from build123d import *

# Parameters (mm, degrees)
EXTRUDE_1_DEPTH = 3.5
EXTRUDE_2_DEPTH = 0.5
EXTRUDE_3_DEPTH = 0.7
SKETCH_4_R      = 2.25
EXTRUDE_4_DEPTH = 0.3
EXTRUDE_5_DEPTH = 1


with BuildPart() as part:
    # 草图1 → 凸台-拉伸1 (new body)
    with BuildSketch(Plane(origin=(0, 0, 0), x_dir=(1, 0, 0), z_dir=(0, 1, 0))):
        Polygon((0, 4.902463921), (0, 1.097536079), (0.55, 0.547536079), (1.097536079, 0), (4.902463921, 0), (5.45, 0.547536079), (6, 1.097536079), (6, 4.902463921), (5.45, 5.452463921), (4.902463921, 6), (1.097536079, 6), (0.55, 5.452463921), align=None)
    extrude(amount=EXTRUDE_1_DEPTH)

    # 草图2 → 凸台-拉伸2 (add)
    with BuildSketch(Plane(origin=(0, 3.5, 0), x_dir=(1, 0, 0), z_dir=(0, 1, 0))):
        Polygon((1.30464286, 5.5), (4.69535714, 5.5), (5.5, 4.69535714), (5.5, 1.30464286), (4.69535714, 0.5), (1.30464286, 0.5), (0.5, 1.30464286), (0.5, 4.69535714), align=None)
    extrude(amount=EXTRUDE_2_DEPTH)

    # 草图3 → 凸台-拉伸3 (add)
    with BuildSketch(Plane(origin=(0, 4, 0), x_dir=(1, 0, 0), z_dir=(0, 1, 0))):
        Polygon((4.591803749, 5.25), (1.408196251, 5.25), (0.75, 4.591803749), (0.75, 1.408196251), (1.408196251, 0.75), (4.591803749, 0.75), (5.25, 1.408196251), (5.25, 4.591803749), align=None)
    extrude(amount=EXTRUDE_3_DEPTH)

    # 草图4 → 凸台-拉伸4 (add)
    with BuildSketch(Plane(origin=(0, 4.7, 0), x_dir=(1, 0, 0), z_dir=(0, 1, 0))):
        with Locations(Location((3, 3, 0), (0, 0, 270))):
            Circle(SKETCH_4_R)
    extrude(amount=EXTRUDE_4_DEPTH)

    # 放样2: read off the stored shape, not the designer's step
    # 放样2: loft between two sections, ruled curve by curve
    loft_2_from = [
        Edge.make_line((1.408196251, 4.7, -5.25), (0.75, 4.7, -4.591803749)),
        Edge.make_line((5.25, 4.7, -4.591803749), (4.591803749, 4.7, -5.25)),
        Edge.make_line((4.591803749, 4.7, -0.75), (5.25, 4.7, -1.408196251)),
        Edge.make_line((0.75, 4.7, -1.408196251), (1.408196251, 4.7, -0.75)),
        Edge.make_line((4.591803749, 4.7, -5.25), (1.408196251, 4.7, -5.25)),
        Edge.make_line((5.25, 4.7, -1.408196251), (5.25, 4.7, -4.591803749)),
        Edge.make_line((0.75, 4.7, -1.408196251), (0.75, 4.7, -4.591803749)),
        Edge.make_line((1.408196251, 4.7, -0.75), (4.591803749, 4.7, -0.75)),
    ]
    loft_2_to = [
        Edge.make_line((1.30464286, 4, -5.5), (0.5, 4, -4.69535714)),
        Edge.make_line((5.5, 4, -4.69535714), (4.69535714, 4, -5.5)),
        Edge.make_line((4.69535714, 4, -0.5), (5.5, 4, -1.30464286)),
        Edge.make_line((0.5, 4, -1.30464286), (1.30464286, 4, -0.5)),
        Edge.make_line((4.69535714, 4, -5.5), (1.30464286, 4, -5.5)),
        Edge.make_line((5.5, 4, -1.30464286), (5.5, 4, -4.69535714)),
        Edge.make_line((0.5, 4, -1.30464286), (0.5, 4, -4.69535714)),
        Edge.make_line((1.30464286, 4, -0.5), (4.69535714, 4, -0.5)),
    ]
    loft_2 = Solid(Shell([*[Face.make_surface_from_curves(loft_2_from[k], loft_2_to[k]) for k in range(8)], Face(Wire(loft_2_from)), Face(Wire(loft_2_to))]))
    add(loft_2)

    # 草图5 → 凸台-拉伸5 (add)
    with BuildSketch(Plane.XZ):
        Polygon((0, -3), (0, -2.3), (-0.15, -2.3), (-0.15, -3.7), (0, -3.7), align=None)
        Polygon((6, -3), (6, -2.3), (6.15, -2.3), (6.15, -3.7), (6, -3.7), align=None)
    extrude(amount=-EXTRUDE_5_DEPTH)


solid = part.part
The listing builds one solid part. Answer for the finished solid, in the listing's coordinates (mm). A direction names the side the tool comes from. Give positions to 0.01 mm unless a question says otherwise; leave off trailing zeros. Write each loop counter-clockwise with the first axis right and the second up, starting at its lowest first coordinate (ties: lowest second). Pieces come first, ordered by that corner, then holes. Notation, with made-up numbers: (-22, 5) - (-10, 5) arc R24 cw to (-10, 43) - close; hole circle Ø1 at (71.5, 27.25). An arc over 180 degrees is marked (long way). Use a Markdown table: item, result.
1. A tool of negligible diameter and unlimited length cuts with its end or side. For faces 1 (the flat face through (0.908, 3.746, -0.897)), 2 (the flat face through (3.2, 3.5, -0.3)), 3 (the flat face through (4.7, 4.7, -4.8)), from which of +Z, -Z, +X, -X, +Y, -Y can it reach the whole face along a straight path? Write none if from no direction.
Values follow:
| item | result |
|---|---|
| face 1 | +Z, -X, +Y |
| face 2 | +Y |
| face 3 | -Z, +X, +Y |
2. Section B-B on x = 5.75 is taken. Write down the section's boundary in (y, z), plus the area to 3 significant figures.
Values follow:
| item | result |
|---|---|
| outline | (0, -5.15) - (3.5, -5.15) - (3.5, -0.85) - (0, -0.85) - close |
| area | 15.1 mm² |
3. This flat-tipped pin is pushed along its axis until it touches: P1, Ø3, axis at y = 3, z = -2, coming from the +X side. Where does it stop, or does it pass through?
Values follow:
| item | result |
|---|---|
| P1 | stops at x = 6 |
4. Find the intervals of material crossed by probe 1 along X at (y, z) = (3.7, -2.55); probe 2 along Y at (x, z) = (1.25, -4.6); probe 3 along X at (y, z) = (2.5, -4.45), in increasing order. Write a range as from..to.
Values follow:
| item | result |
|---|---|
| probe 1 | x = 0.5..5.5 |
| probe 2 | y = 0..4.7 |
| probe 3 | x = 0..6 |
5. Section A-A on y = 3.35 is taken. Write down the section's boundary in (x, z).
Values follow:
| item | result |
|---|---|
| outline | (0, -4.9) - (1.1, -6) - (4.9, -6) - (6, -4.9) - (6, -1.1) - (4.9, 0) - (1.1, 0) - (0, -1.1) - close |
